Read the model definition and answer for the solid it produces. Units are mm, in the model's axes. A direction names the side the tool comes from. Round coordinates to 2 decimals unless told otherwise and drop trailing zeros. Write each loop counter-clockwise with the first axis right and the second up, starting at its lowest first coordinate (ties: lowest second). Pieces come first, ordered by that corner, then holes.
from build123d import *

# Parameters (mm, degrees)
SKETCH1_R           = 8.5
BOSS_EXTRUDE1_DEPTH = 5.5
SKETCH2_R           = 2.485
BOSS_EXTRUDE2_DEPTH = 13.5
CHAMFER1_SIZE       = 0.5
SKETCH5_R           = 4.5
CUT_EXTRUDE3_DEPTH  = 2.54
SKETCH3_R           = 2.04
CUT_EXTRUDE1_DEPTH  = 2.35
SKETCH4_R           = 1.065
CUT_EXTRUDE2_DEPTH  = 22.35
SKETCH7_R           = 5
CUT_EXTRUDE5_DEPTH  = 11.54
CIRPATTERN1_COUNT   = 3


with BuildPart() as part:
    # Sketch1 → Boss-Extrude1 (new body)
    with BuildSketch(Plane(origin=(0, 0, 0), x_dir=(1, 0, 0), z_dir=(0, 1, 0))):
        with Locations(Location((0, 0, 0), (0, 0, 270))):
            Circle(SKETCH1_R)
    extrude(amount=BOSS_EXTRUDE1_DEPTH)

    # Sketch2 → Boss-Extrude2 (add)
    with BuildSketch(Plane(origin=(0, 5.5, 0), x_dir=(1, 0, 0), z_dir=(0, 1, 0))):
        with Locations(Location((0, 0, 0), (0, 0, 270))):
            Circle(SKETCH2_R)
    extrude(amount=BOSS_EXTRUDE2_DEPTH)

    # Chamfer1
    chamfer1_edges = [part.edges().sort_by_distance(p)[0] for p in [
        (0, 19, -2.485),
    ]]
    chamfer(chamfer1_edges, length=CHAMFER1_SIZE)

    # Sketch5 → Cut-Extrude3 (cut)
    with BuildSketch(Plane.XZ):
        with Locations(Location((0, 0, 0), (0, 0, 270))):
            Circle(SKETCH5_R)
    extrude(amount=-CUT_EXTRUDE3_DEPTH, mode=Mode.SUBTRACT)

    # Sketch3 → Cut-Extrude1 (cut)
    with BuildSketch(Plane(origin=(0, 5.5, 0), x_dir=(1, 0, 0), z_dir=(0, 1, 0))):
        with Locations(Location((0, 5.773502692, 0), (0, 0, 270))):
            Circle(SKETCH3_R)
        with Locations(Location((5, -2.886751346, 0), (0, 0, 270))):
            Circle(SKETCH3_R)
        with Locations(Location((-5, -2.886751346, 0), (0, 0, 270))):
            Circle(SKETCH3_R)
    extrude(amount=-CUT_EXTRUDE1_DEPTH, mode=Mode.SUBTRACT)

    # Sketch4 → Cut-Extrude2 (cut)
    with BuildSketch(Plane(origin=(0, 3.15, 0), x_dir=(1, 0, 0), z_dir=(0, 1, 0))):
        with Locations(Location((0, 5.773502692, 0), (0, 0, 270))):
            Circle(SKETCH4_R)
        with Locations(Location((5, -2.886751346, 0), (0, 0, 270))):
            Circle(SKETCH4_R)
        with Locations(Location((-5, -2.886751346, 0), (0, 0, 270))):
            Circle(SKETCH4_R)
    extrude(amount=-CUT_EXTRUDE2_DEPTH, mode=Mode.SUBTRACT)

    # Sketch7 → Cut-Extrude5 (cut)
    with BuildSketch(Plane(origin=(0, 2.474873734, 2.474873734), x_dir=(1, 0, 0), z_dir=(0, 0.7071067811865476, 0.7071067811865476))):
        with Locations((0, -8.121320344)):
            Circle(SKETCH7_R)
    cut_extrude5 = extrude(amount=CUT_EXTRUDE5_DEPTH, mode=Mode.SUBTRACT)

    # CirPattern1: Cut-Extrude5 ×3 about axis
    cirpattern1_axis = Axis((0, 0, 0), (0, 1, 0))
    for i in range(1, CIRPATTERN1_COUNT):
        add(cut_extrude5.rotate(cirpattern1_axis, i * 360 / CIRPATTERN1_COUNT), mode=Mode.SUBTRACT)


solid = part.part
Q1. Which of the six approach directions +Z, -Z, +X, -X, +Y, -Y give full straight-line access (tool end or side, diameter ignored) to faces 1 (the cylindrical face through (1.352, 1.252, -4.292)), 2 (the flat face through (4.4, 0, -1.7)), 3 (the cylindrical face through (4.22, 4.34, 4.77))?
Verdict:
face 1: -Y
face 2: +Z, -Z, +X, -X, -Y
face 3: +Y
Q2. Section B-B (y = 14.25) is taken. Determine the outline of the cut face in (x, z) (3 decimals), then the cut area to 3 significant figures.
Verdict:
outline: circle Ø4.97 at (0, 0)
area: 19.4 mm2
Q3. Flat-ended cylindrical pins translate along their axes: pin 1 Ø3 at (x, z) = (4, 1.5) entering from +Y; pin 2 Ø4.5 at (x, z) = (0.5, -1.5) entering from -Y; pin 3 Ø1 at (y, z) = (5.5, 3.5) entering from +X; pin 4 Ø1.7 at (x, z) = (-5, 2.89) entering from -Y. Find the tip coordinate at first contact, or state that the pin passes through.
Verdict:
pin 1: stops at y = 5.5
pin 2: stops at y = 2.54
pin 3: stops at x = 7.95
pin 4: passes through
Q4. Determine the mould class of faces 4 (the cylindrical face through (2.55, 3.32, 8.11)), 5 (the flat face through (0, 2.54, 0)), 6 (the flat face through (-2, 5.5, 2)) for opening direction Z: pulls with the +Z half, pulls with the -Z half, needs draft (parallel to the pull), parting line crosses it, or undercut.
Verdict:
face 4: parting line crosses it
face 5: undercut
face 6: needs draft
Q5. Straight lines are drawn through the part: probe 1 along Y at (x, z) = (-4, 0); probe 2 along X at (y, z) = (2, -0.5); probe 3 along Y at (x, z) = (6.5, 4.5). For each, find the intervals that lie inside material, in ascending order.
Verdict:
probe 1: y = 2.54 to 5.5
probe 2: x = -8.49 to -4.47, 4.47 to 8.49
probe 3: y = 0 to 5.5
